The listing builds one solid part. Answer for the finished solid, in the listing's coordinates (mm). A direction names the side the tool comes from. Round coordinates to 2 decimals unless told otherwise and drop trailing zeros. Write each loop counter-clockwise with the first axis right and the second up, starting at its lowest first coordinate (ties: lowest second). Pieces come first, ordered by that corner, then holes. Notation, with made-up numbers: M 87,-9.5 L 120,-9.5 A10 ccw 120,7.5 Z; hole C -40,-14 d7. An arc over 180 degrees is marked long. Write each question's results on one line, items separated by ' | '.
Autodesk Inventor part; units mm, degrees
ref_plane "YZ Plane" through (0, 0, 0) normal (1, 0, 0) x (0, 1, 0)
ref_plane "XZ Plane" through (0, 0, 0) normal (0, 1, 0) x (-1, 0, 0)
ref_plane "XY Plane" through (0, 0, 0) normal (0, 0, 1) x (1, 0, 0)
sketch "Sketch1" plane through (0, 0, 0) normal (0, 1, 0) x (-1, 0, 0)
  line L0 (25.6659, 82.3437) -> (46.406, 61.6036)
  line L1 (46.406, 61.6036) -> (46.406, 8.9397)
  circle A0 centre (23.593, 50.6893) radius 1.75
  circle A1 centre (23.593, 50.6893) radius 1.75
  line L2 (46.406, 8.9397) -> (26.093, 8.9397)
  line L3 (26.093, 47) -> (19.9037, 47)
  line L4 (19.9037, 47) -> (19.9037, 59.379)
  line L5 (11.3025, 67.9802) -> (19.9037, 59.379)
  line L6 (26.093, 47) -> (26.093, 8.9397)
  line L7 (25.6659, 82.3437) -> (11.3025, 67.9802)
extrude "Extrusion3" add sketch "Sketch1" along normal blind 2
sketch "Sketch3" plane through (0, 2, 0) normal (0, 1, 0) x (1, 0, 0)
  circle A0 centre (-23.593, -50.6893) radius 1.75
  line L0 (-46.406, -8.9397) -> (-46.406, -61.6036)
  line L1 (-46.406, -61.6036) -> (-25.6659, -82.3437)
  line L2 (-25.6659, -82.3437) -> (-11.3025, -67.9802)
  line L3 (-11.3025, -67.9802) -> (-19.9037, -59.379)
  line L4 (-19.9037, -59.379) -> (-19.9037, -47)
  line L5 (-19.9037, -47) -> (-26.093, -47)
  line L6 (-26.093, -47) -> (-26.093, -8.9397)
  line L7 (-26.093, -8.9397) -> (-46.406, -8.9397)
  line L8 (-46.406, -8.9397) -> (-46.406, -23.9397)
  line L9 (-46.406, -23.9397) -> (-44.406, -23.9397)
  line L10 (-44.406, -23.9397) -> (-44.406, -8.9397)
  line L11 (-44.406, -8.9397) -> (-46.406, -8.9397)
  line L12 (-46.406, -8.9397) -> (-31.406, -8.9397) construction
  line L13 (-46.406, -61.6036) -> (-46.406, -46.6036)
  line L14 (-46.406, -46.6036) -> (-44.406, -46.6036)
  line L15 (-44.406, -46.6036) -> (-44.406, -61.6036)
  line L16 (-44.406, -61.6036) -> (-46.406, -61.6036)
  line L17 (-46.406, -61.6036) -> (-31.406, -61.6036) construction
  line L18 (-46.406, -61.6036) -> (-35.7994, -72.2102)
  line L19 (-35.7994, -72.2102) -> (-34.3852, -70.796)
  line L20 (-34.3852, -70.796) -> (-44.9918, -60.1894)
  line L21 (-44.9918, -60.1894) -> (-46.406, -61.6036)
  line L22 (-46.406, -61.6036) -> (-31.406, -61.6036) construction
  line L23 (-46.406, -61.6036) -> (-25.6659, -82.3437)
  line L24 (-25.6659, -82.3437) -> (-30.9692, -77.0404)
  line L25 (-30.9692, -77.0404) -> (-29.555, -75.6262)
  line L26 (-29.555, -75.6262) -> (-24.2517, -80.9295)
  line L27 (-24.2517, -80.9295) -> (-25.6659, -82.3437)
  point P0 (0, 0)
  dimension "d20" = 15
  dimension "d21" = 90
  dimension "d22" = 2
  dimension "d23" = 15
  dimension "d24" = 90
  dimension "d25" = 2
  dimension "d26" = 15
  dimension "d27" = 45
  dimension "d28" = 2
  dimension "d29" = 7.5
  dimension "d30" = 2
extrude "Extrusion4" add sketch "Sketch3" along normal blind 15 contours L7 L10 L9 L0 | L14 L15 L20 L21 L0 | L16 L15 L20 L19 L1 | L21 L20 L15 L16 | L25 L26 L2 L1
properties part number "covfronti2c2"
1) The mould has two halves that part along Z. Classify faces 6 (the face through (-23.214, 0.986, 52.398)), 7 (the face through (-35.1, 9.4, 71.51)), 8 (the face through (-45, 17, 60)): +Z half, -Z half, draft (parallel to the pull), parting line (faces both ways), or undercut.
Return value:
face 6: undercut | face 7: +Z half | face 8: draft
2) Each of these flat-tipped pins is pushed along its axis until it touches: pin 1 (3 mm diameter, centred on x = -37, z = 52.5, fed in from +Y); pin 2 (12 mm diameter, centred on x = -40, z = 66.5, fed in from -Y); pin 3 (1 mm diameter, centred on x = -23, y = 1, fed in from -Z); pin 4 (1.5 mm diameter, centred on x = -36, y = 14.5, fed in from -Z). Where does it stop, or does it pass through?
Return value:
pin 1: y = 2 | pin 2: y = 0 | pin 3: z = 47 | pin 4: z = 68.43
3) Section D-D (z = 26.5) is taken. Determine the outline of the cut face in (x, y).
Return value:
outline: M -46.41,0 L -26.09,0 L -26.09,2 L -46.41,2 Z
4) A tool of negligible diameter and unlimited length cuts with its end or side. For faces 1 (the face through (-19.904, 1, 53)), 2 (the face through (-21.71, 1.53, 78.39)), 3 (the face through (-30.27, 9.4, 76.34)), 4 (the face through (-39.325, 9.395, 65.856)), 5 (the face through (-45, 9, 23.94)), from which of +Z, -Z, +X, -X, +Y, -Y can it reach the whole face along a straight path? Write none if from no direction.
Return value:
face 1: -Z, +X, +Y, -Y | face 2: +Z, +X, +Y, -Y | face 3: -Z, -X, +Y | face 4: -Z, +X, +Y | face 5: +X, -X, +Y
5) Section C-C (x = -43) is taken. Determine the outline of the cut face in (y, z), then the cut area to 3 significant figures.
Return value:
outline: M 0,8.94 L 2,8.94 L 2,62.18 L 17,62.18 L 17,65.01 L 0,65.01 Z | area: 155 mm²
6) Section B-B (z = 17) is taken. Determine the outline of the cut face in (x, y), then the cut area to 3 significant figures.
Return value:
outline: M -46.41,0 L -26.09,0 L -26.09,2 L -44.41,2 L -44.41,17 L -46.41,17 Z | area: 70.6 mm²
7) Section A-A (y = 9.25) is taken. Determine the outline of the cut face in (x, z) (1 decimal).
Return value:
outline: M -46.4,8.9 L -44.4,8.9 L -44.4,23.9 L -46.4,23.9 Z; M -46.4,46.6 L -44.4,46.6 L -44.4,60.8 L -34.4,70.8 L -35.8,72.2 L -46.4,61.6 Z; M -31,77 L -29.6,75.6 L -24.3,80.9 L -25.7,82.3 Z
8) Find the intervals of material crossed by line 1 (Y direction, x = -32.5, z = 68.5); line 2 (X direction, y = 3, z = 21); line 3 (Z direction, x = -24, y = 1.5), in increasing order.
Return value:
line 1: 0 to 2 | line 2: -46.41 to -44.41 | line 3: 47 to 48.99, 52.39 to 80.68
